Here's how the part is built. I have some questions about the finished solid (model axes, mm). Face numbers are marked on the shaded views. A direction names the side the tool comes from. Give positions to 0.01 mm unless a question says otherwise; leave off trailing zeros. Loops run counter-clockwise (first coordinate to the right, second up) from the corner with the lowest first, then second, coordinate; pieces in that order, holes last. Notation, with made-up numbers: (77, 26) -> (113, 26) arc R23 ccw to (113, 47) -> close; hole circle Ø4 at (65.25, -38.5). An arc over 180 degrees is marked (long way). Answer in a Markdown table with one row per item. Add a question column.
Item 1: If we section it at A-A (z = 5): Write out the boundary of the cut face in (x, y), then the cut area to 3 significant figures.
Item 2: We'd pull the mould along Z, two halves only. Please class the marked faces 1, 2 and 3: released by +Z, released by -Z, zero draft, split by the parting line, or undercut.
Item 3: If we section it at B-B (x = 18.5): Write out the boundary of the cut face in (y, z).
Item 4: If we section it at C-C (y = -10.5): Write out the boundary of the cut face in (x, z).
Item 5: Which directions (+Z, -Z, +X, -X, +Y, -Y) give clear straight access to the entire face, cutting with the end or side of a thin tool? Please do the marked faces 4 and 5.
Item 6: If I drill on line 1 (Z direction, x = 0, y = 10); line 2 (X direction, y = 16.5, z = 1.5); line 3 (X direction, y = -11, z = -5.5), over which ranges is the centre line in solid material (lowest first)?
Item 7: For P1, Ø2, axis at x = 14.5, z = 0, coming from the +Y side; P2, Ø8.5, axis at x = 12, z = -1.5, coming from the -Y side; P3, Ø4, axis at y = 10.5, z = 2, coming from the +X side, each with a flat end and sliding along its axis, tell me the tip position at first contact or that it passes through.
```python
from build123d import *

# Parameters (mm, degrees)
BOSS_EXTRU_1_DEPTH                  = 10
ENL_V_START                         = 0.5
ESQUISSE3_W                         = 17
ESQUISSE3_H                         = 125.217180483
ENL_V_MAT_EXTRU_2_DEPTH             = 20
ENL_V_MAT_EXTRU_3_REACH             = 41.835
DIAM_TRE_DU_PER_AGE_5_0_5_2_D       = 5
DIAM_TRE_DU_PER_AGE_1_5_1_5_1_D     = 1.5
DIAM_TRE_DU_PER_AGE_1_5_1_5_1_DEPTH = 5
DIAM_TRE_DU_PER_AGE_1_5_1_5_1_TIP   = 0.450645464


with BuildPart() as part:
    # Esquisse1 → Boss.-Extru.1 (new body, symmetric)
    with BuildSketch(Plane.XY):
        Polygon((85.767026828, -38.334571354), (88.53088082, -34.167904687), (0, 35), (-15.366750419, 35), (-22, 25), (-22, 13), align=None)
    extrude(amount=BOSS_EXTRU_1_DEPTH, both=True)

    # Esquisse3 → Enlèv. mat.-Extru.2 (cut)
    with BuildSketch(Plane(origin=(5.827214604, 9.698113705, 0), x_dir=(0, 0, -1), z_dir=(0.515038075, 0.857167301, 0)).offset(ENL_V_START)):
        with Locations((0, -30.874957754)):
            Rectangle(ESQUISSE3_W, ESQUISSE3_H)
    extrude(amount=ENL_V_MAT_EXTRU_2_DEPTH, mode=Mode.SUBTRACT)

    # Esquisse4 → Enlèv. mat.-Extru.3 (cut, up to next)
    with BuildSketch(Plane(origin=(0, 1.5, 0), x_dir=(1, 0, 0), z_dir=(0, 1, 0)), mode=Mode.PRIVATE) as enl_v_mat_extru_3_sk1:
        with BuildLine():
            Line((0.413793103, 3.978539338), (14.75862069, 2.486587087))
            ThreePointArc((14.75862069, 2.486587087), (17, 0), (14.75862069, -2.486587087))
            Line((14.75862069, -2.486587087), (0.413793103, -3.978539338))
            ThreePointArc((0.413793103, -3.978539338), (-4, 0), (0.413793103, 3.978539338))
        make_face()
    enl_v_mat_extru_3_tool1 = extrude(enl_v_mat_extru_3_sk1.sketch, amount=-ENL_V_MAT_EXTRU_3_REACH, mode=Mode.PRIVATE) & part.part
    add(enl_v_mat_extru_3_tool1.solids().sort_by_distance((5.738323, 1.5, 0))[0], mode=Mode.SUBTRACT)

    # Diamètre du perçage Ø5.0 (5)2 (through all)
    with Locations(Plane(origin=(0, 1.5, 0), x_dir=(-1, 0, 0), z_dir=(0, -1, 0))):
        with Locations((0, 0)):
            Hole(DIAM_TRE_DU_PER_AGE_5_0_5_2_D / 2)

    # Diamètre du perçage Ø1.5 (1.5)1
    with Locations(Plane(origin=(0, 1.5, 0), x_dir=(-1, 0, 0), z_dir=(0, -1, 0))):
        with Locations((-14.5, 0), (-4.5, 0)):
            Hole(DIAM_TRE_DU_PER_AGE_1_5_1_5_1_D / 2, depth=DIAM_TRE_DU_PER_AGE_1_5_1_5_1_DEPTH)
            with Locations((0, 0, -(DIAM_TRE_DU_PER_AGE_1_5_1_5_1_DEPTH + DIAM_TRE_DU_PER_AGE_1_5_1_5_1_TIP / 2))):  # 118° drill point
                Cone(0, DIAM_TRE_DU_PER_AGE_1_5_1_5_1_D / 2, DIAM_TRE_DU_PER_AGE_1_5_1_5_1_TIP, mode=Mode.SUBTRACT)


solid = part.part
```
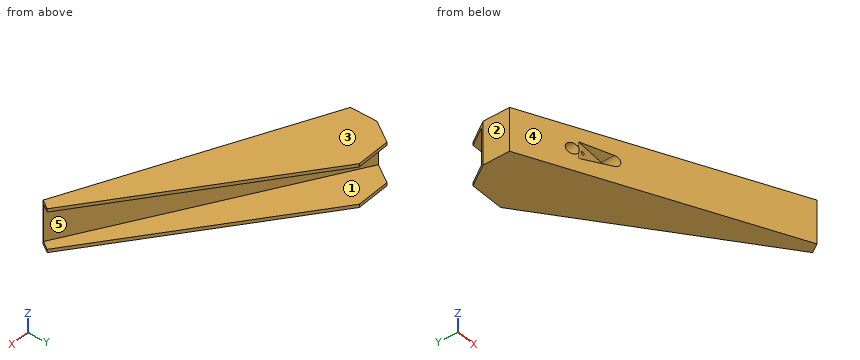
Recorded:
| question | item | result |
|---|---|---|
| 1 | outline | (-22, 13) -> (85.77, -38.33) -> (86.04, -37.92) -> (-21.05, 26.43) -> (-22, 25) -> close |
| 1 | area | 785 mm^2 |
| 2 | face 1 | undercut |
| 2 | face 2 | zero draft |
| 2 | face 3 | released by +Z |
| 3 | outline | (-6.29, -10) -> (20.55, -10) -> (20.55, -8.5) -> (2.67, -8.5) -> (2.67, 8.5) -> (20.55, 8.5) -> (20.55, 10) -> (-6.29, 10) -> close |
| 4 | outline | (27.33, -10) -> (58.24, -10) -> (58.24, -8.5) -> (40.41, -8.5) -> (40.41, 8.5) -> (58.24, 8.5) -> (58.24, 10) -> (27.33, 10) -> close |
| 5 | face 4 | +Z, -Z, -X, -Y |
| 5 | face 5 | +X, +Y |
| 6 | line 1 | z = -10 to -2.5, 2.5 to 10 |
| 6 | line 2 | x = -22 to -4.52 |
| 6 | line 3 | x = 28.38 to 41.25 |
| 7 | P1 | stops at y = 5.67 |
| 7 | P2 | stops at y = -5.22 |
| 7 | P3 | stops at x = 8.79 |
